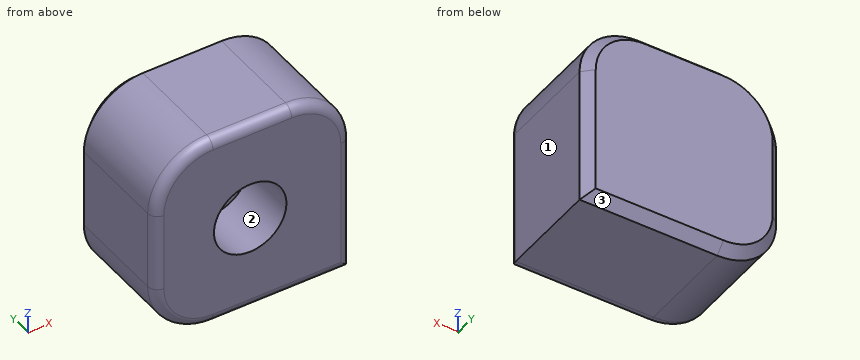
```python
from build123d import *

# Parameters (mm, degrees)
F1_DEPTH = 60
F2_R     = 5
F3_SIZE  = 5
F4_R     = 18.436083
F5_DEPTH = 30


with BuildPart() as f1:
    # F0 (on Front) → F1 (new body)
    with BuildSketch(Plane.XZ):
        with BuildLine():
            Line((21.084471, 76.11473), (-18.915529, 76.11473))
            ThreePointArc((-18.915529, 76.11473), (-40.128732, 67.327933), (-48.915529, 46.11473))
            Line((-48.915529, 46.11473), (-48.915529, 6.11473))
            ThreePointArc((-48.915529, 6.11473), (-40.128732, -15.098474), (-18.915529, -23.88527))
            Line((-18.915529, -23.88527), (51.084471, -23.88527))
            Line((51.084471, -23.88527), (51.084471, 46.11473))
            ThreePointArc((51.084471, 46.11473), (42.297675, 67.327933), (21.084471, 76.11473))
        make_face()
    extrude(amount=F1_DEPTH)

    # F2
    f2_edges = [f1.edges().sort_by_distance(p)[0] for p in [
        (51.084471, -60, 11.11473),
        (42.297675, -60, 67.327933),
        (1.084471, -60, 76.11473),
        (-40.128732, -60, 67.327933),
        (-48.915529, -60, 26.11473),
        (-40.128732, -60, -15.098474),
        (16.084471, -60, -23.88527),
    ]]
    fillet(f2_edges, radius=F2_R)

    # F3
    f3_edges = [f1.edges().sort_by_distance(p)[0] for p in [
        (51.084471, 0, 11.11473),
        (42.297675, 0, 67.327933),
        (1.084471, 0, 76.11473),
        (-40.128732, 0, 67.327933),
        (-48.915529, 0, 26.11473),
        (-40.128732, 0, -15.098474),
        (16.084471, 0, -23.88527),
    ]]
    chamfer(f3_edges, length=F3_SIZE)

    # F4 (on face) → F5 (cut)
    with BuildSketch(Plane.XZ.offset(60)):
        with Locations((0, 25.528846)):
            Circle(F4_R)
    extrude(amount=-F5_DEPTH, mode=Mode.SUBTRACT)


solid = f1.part
```
Build history of the part. All positions in model axes, mm. Face numbers are marked on the shaded views. Round coordinates to 2 decimals unless told otherwise and drop trailing zeros. Write each loop counter-clockwise with the first axis right and the second up, starting at its lowest first coordinate (ties: lowest second). Pieces come first, ordered by that corner, then holes. Notation, with made-up numbers: (34, 89) - (71, 89) arc R19 ccw to (71, 105) - close; hole circle Ø4 at (-35.5, 2). An arc over 180 degrees is marked (long way). Write each question's results on one line, items separated by ' | '. Start each with the question number.
Item 1: Drop flat-ended pins along their axis: P1, Ø1.5, axis at x = 9.5, z = 11.5, coming from the -Y side; P2, Ø5, axis at x = -23, y = -33.5, coming from the -Z side; P3, Ø10, axis at y = -15, z = 64, coming from the -X side. Give the stop position or say it passes through.
Item 2: Wall check: L1, parallel to Z at x = 0, y = -52; L2, parallel to X at y = -46, z = 21; L3, parallel to Y at x = -3.5, z = 36. Give the ranges that are in metal, low to high. Write a range as [from, to].
Item 3: Saw through at C-C (z = 20). Write the cut outline in (x, y), and give its area (3 significant figures).
Item 4: Saw through at B-B (y = -42). Write the cut outline in (x, z), and give its area (3 significant figures).
Item 5: Saw through at D-D (y = -8). Write the cut outline in (x, z), and give its area (3 significant figures).
Item 6: Mould opens along Z. For the marked faces 1, 2 and 3 say: pulls with the +Z half, pulls with the -Z half, needs draft (parallel to the pull), parting line crosses it, or undercut.
Item 7: Saw through at A-A (x = 0). Write the cut outline in (y, z).
Results are:
1) P1: stops at y = -30 | P2: stops at z = -23.84 | P3: stops at x = -46.01
2) L1: z = [-23.89, 7.09], [43.96, 76.11] | L2: x = [-48.92, -17.87], [17.87, 51.08] | L3: y = [-30, 0]
3) outline: (-48.92, -55) arc R5 ccw to (-43.92, -60) - (-17.59, -60) - (-17.59, -30) - (17.59, -30) - (17.59, -60) - (46.08, -60) arc R5 ccw to (51.08, -55) - (51.08, -5) - (46.08, 0) - (-43.92, 0) - (-48.92, -5) - close | area: 4,910 mm²
4) outline: (-48.92, 6.11) arc R30 ccw to (-18.92, -23.89) - (51.08, -23.89) - (51.08, 46.11) arc R30 ccw to (21.08, 76.11) - (-18.92, 76.11) arc R30 ccw to (-48.92, 46.11) - close; hole circle Ø36.87 at (0, 25.53) | area: 8,350 mm²
5) outline: (-48.92, 6.11) arc R30 ccw to (-18.92, -23.89) - (51.08, -23.89) - (51.08, 46.11) arc R30 ccw to (21.08, 76.11) - (-18.92, 76.11) arc R30 ccw to (-48.92, 46.11) - close | area: 9,420 mm²
6) face 1: needs draft | face 2: undercut | face 3: pulls with the -Z half
7) outline: (-60, -18.89) arc R5 ccw to (-55, -23.89) - (-5, -23.89) - (0, -18.89) - (0, 71.11) - (-5, 76.11) - (-55, 76.11) arc R5 ccw to (-60, 71.11) - (-60, 43.96) - (-30, 43.96) - (-30, 7.09) - (-60, 7.09) - close
